Work out the finished part from the listing and answer in its coordinate system (mm). A direction names the side the tool comes from. Round coordinates to 2 decimals unless told otherwise and drop trailing zeros. Write each loop counter-clockwise with the first axis right and the second up, starting at its lowest first coordinate (ties: lowest second). Pieces come first, ordered by that corner, then holes. Notation, with made-up numbers: M 76,49 L 91,49 A9 ccw 91,54 Z; hole C -8.5,57.5 d3. An arc over 180 degrees is marked long. Answer in a Markdown table with one row per item.
```python
from build123d import *

# Parameters (mm, degrees)
SKETCH1_W               = 86.4
SKETCH1_H               = 25
BOSS_EXTRUDE1_DEPTH     = 3
CUT_EXTRUDE2_DEPTH      = 58.935016495
CUT_EXTRUDE2_DEPTH_BACK = 58.935016495
SKETCH2_R               = 2
FILLET1_R               = 2


with BuildPart() as part:
    # Sketch1 → Boss-Extrude1 (new body)
    with BuildSketch(Plane.XY):
        Polygon((-50.636338419, 24.154507628), (-50.636338419, 18.154507628), (-50.636338419, 16.154507628), (-50.636338419, -25.845492372), (51.763661581, -25.845492372), (51.763661581, 16.154507628), (51.763661581, 18.154507628), (51.763661581, 24.154507628), align=None)
        with Locations((0.563661581, -3.345492372)):
            Rectangle(SKETCH1_W, SKETCH1_H, mode=Mode.SUBTRACT)
    extrude(amount=BOSS_EXTRUDE1_DEPTH)

    # Sketch2 → Cut-Extrude2 (cut, two sides: drawn at the far end of the back side and taken through both)
    with BuildSketch(Plane.XY.offset(3).offset(-CUT_EXTRUDE2_DEPTH_BACK)):
        with Locations((-29.436338419, 20.154507628)):
            Circle(SKETCH2_R)
        with Locations((-29.436338419, -20.845492372)):
            Circle(SKETCH2_R)
        with Locations((-9.436338419, -20.845492372)):
            Circle(SKETCH2_R)
        with Locations((-9.436338419, 20.154507628)):
            Circle(SKETCH2_R)
        with Locations((10.563661581, -20.845492372)):
            Circle(SKETCH2_R)
        with Locations((10.563661581, 20.154507628)):
            Circle(SKETCH2_R)
        with Locations((30.563661581, -20.845492372)):
            Circle(SKETCH2_R)
        with Locations((30.563661581, 20.154507628)):
            Circle(SKETCH2_R)
    extrude(amount=CUT_EXTRUDE2_DEPTH + CUT_EXTRUDE2_DEPTH_BACK, mode=Mode.SUBTRACT)

    # Fillet1
    fillet1_edges = [part.edges().sort_by_distance(p)[0] for p in [
        (51.763661581, -25.845492372, 1.5),
        (-50.636338419, -25.845492372, 1.5),
        (-42.636338419, -15.845492372, 1.5),
        (43.763661581, -15.845492372, 1.5),
    ]]
    fillet(fillet1_edges, radius=FILLET1_R)


solid = part.part
```
1. The part is cut by section C-C (x = 30). Determine the outline of the cut face in (y, z).
Calculated:
| item | result |
|---|---|
| outline | M -25.85,0 L -22.76,0 L -22.76,3 L -25.85,3 Z; M -18.93,0 L -15.85,0 L -15.85,3 L -18.93,3 Z; M 9.15,0 L 18.24,0 L 18.24,3 L 9.15,3 Z; M 22.07,0 L 24.15,0 L 24.15,3 L 22.07,3 Z |
2. The part is cut by section A-A (y = -6). Determine the outline of the cut face in (x, z).
Calculated:
| item | result |
|---|---|
| outline | M -50.64,0 L -42.64,0 L -42.64,3 L -50.64,3 Z; M 43.76,0 L 51.76,0 L 51.76,3 L 43.76,3 Z |
3. The part is cut by section B-B (x = -21). Determine the outline of the cut face in (y, z).
Calculated:
| item | result |
|---|---|
| outline | M -25.85,0 L -15.85,0 L -15.85,3 L -25.85,3 Z; M 9.15,0 L 24.15,0 L 24.15,3 L 9.15,3 Z |
4. Given pin 1 (3.5 mm diameter, centred on x = 30.56, y = -20.85, fed in from +Z), flat-ended and moving along its own axis, determine where the tip first touches the part or whether it passes through.
Calculated:
| item | result |
|---|---|
| pin 1 | passes through |
5. A tool of negligible diameter and unlimited length cuts with its end or side. For faces 1 (the flat face through (0, -15.845, 1)), 2 (the flat face through (51.764, 0, 1)), from which of +Z, -Z, +X, -X, +Y, -Y can it reach the whole face along a straight path? Write none if from no direction.
Calculated:
| item | result |
|---|---|
| face 1 | +Z, -Z |
| face 2 | +Z, -Z, +X, +Y, -Y |
6. The part is cut by section D-D (z = 1.6). Count the separate pieces of the cut face and the enclosed holes in it, plus the area to 3 significant figures.
Calculated:
| item | result |
|---|---|
| separate pieces | 1 |
| enclosed holes | 9 |
| area | 2,860 mm² |
7. Consider line 1 along X through (y, z) = (20, 1.9); line 2 along Y through (x, z) = (10.5, 1.3); line 3 along Y through (x, z) = (-11.5, 1.2). Determine where each line is inside the solid, lowest interval first. Write a range as from..to.
Calculated:
| item | result |
|---|---|
| line 1 | x = -50.64..-31.43, -27.44..-11.43, -7.44..8.57, 12.56..28.57, 32.56..51.76 |
| line 2 | y = -25.85..-22.84, -18.85..-15.85, 9.15..18.16, 22.15..24.15 |
| line 3 | y = -25.85..-15.85, 9.15..24.15 |
8. Determine the mould class of faces 3 (the cylindrical face through (51.16, -25.28, 1.52)), 4 (the cylindrical face through (8.977, -22.062, 1.479)), 5 (the flat face through (1, 24.155, 1)), 6 (the flat face through (-50.636, 0, 1)) for opening direction X: released by +X, released by -X, zero draft, split by the parting line, or undercut.
Calculated:
| item | result |
|---|---|
| face 3 | released by +X |
| face 4 | undercut |
| face 5 | zero draft |
| face 6 | released by -X |
